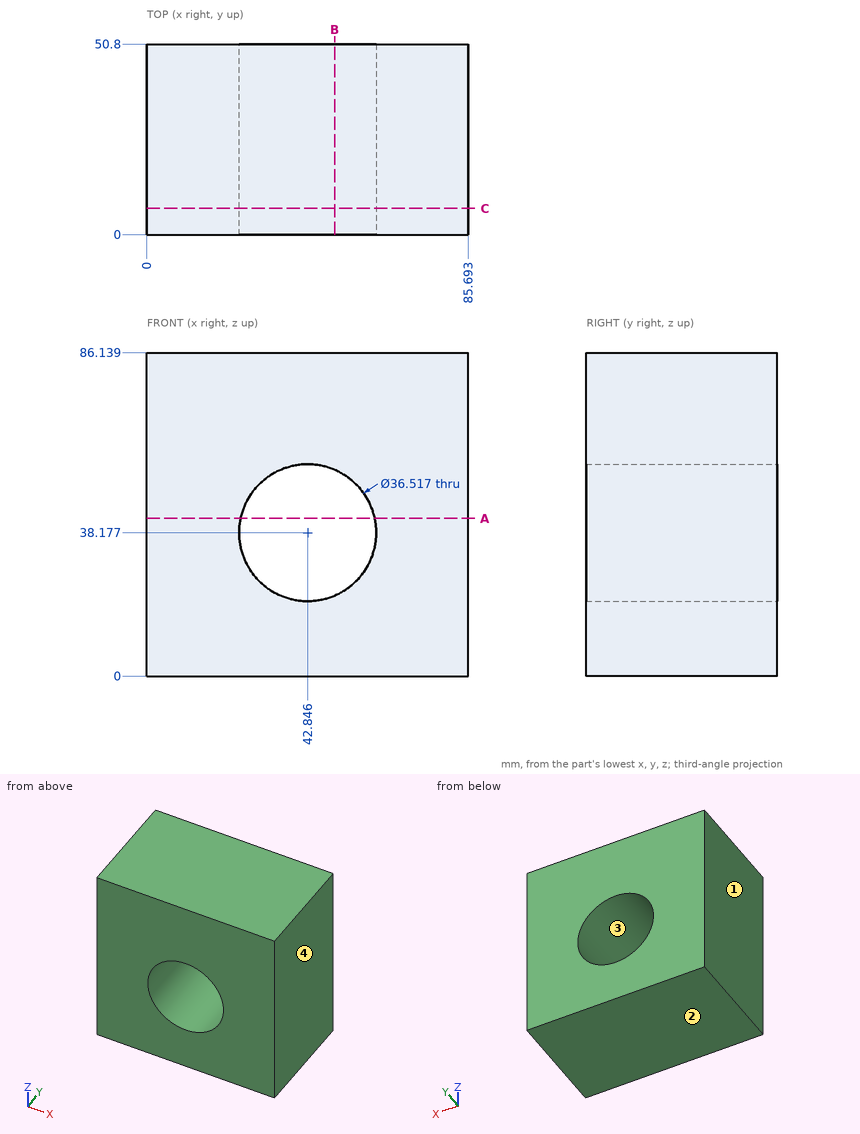
Print and shaded views of the part. All mm, measured from the part's lowest x, y and z. Coordinates: 2 decimals unless noted, no trailing zeros. Loops run counter-clockwise (first coordinate to the right, second up) from the corner with the lowest first, then second, coordinate; pieces in that order, holes last. Notation, with made-up numbers: (17, 24.25) - (21, 24.25) arc R25 cw to (21, 36.25) - close; hole circle Ø3 at (31, 1). An arc over 180 degrees is marked (long way). Use one line per item in the form item = value. Start each with the question number.
1) Two-plate mould, pull along X, no slides. Class the marked faces 1, 2, 3 and 4: +X half, -X half, draft (parallel to the pull), parting line (faces both ways), or undercut.
2) Flat gauge pin, fed straight in: pin 1 (10 mm diameter, centred on x = 37.5, z = 50.5, fed in from +Y). Where does the tip first touch, or does it go through?
3) Band-saw the part on B-B (x = 50). Give the cut face in (y, z) (1 decimal).
4) Band-saw the part on A-A (z = 42). Give the cut face in (x, y).
5) Band-saw the part on C-C (y = 7). Give the cut face in (x, z) (1 decimal), and give its area (3 significant figures).
6) Drill centre lines: L1, parallel to Z at x = 49, y = 20; L2, parallel to Z at x = 32, y = 3 (1 decimal); L3, parallel to X at y = 33, z = 29.5. Where is each one in solid material? Low to high. Write a range as from..to.
Check values:
q1.face_1 = -X half
q1.face_2 = draft
q1.face_3 = undercut
q1.face_4 = +X half
q2.pin_1 = 50.8
q3.outline = (0, 0) - (50.8, 0) - (50.8, 21.4) - (0, 21.4) - close; (0, 55) - (50.8, 55) - (50.8, 86.1) - (0, 86.1) - close
q4.outline = (0, 0) - (24.99, 0) - (24.99, 50.8) - (0, 50.8) - close; (60.7, 0) - (85.69, 0) - (85.69, 50.8) - (60.7, 50.8) - close
q5.outline = (0, 0) - (85.7, 0) - (85.7, 86.1) - (0, 86.1) - close; hole circle Ø36.5 at (42.8, 38.2)
q5.area = 6,330 mm2
q6.L1 = 0..20.99, 55.37..86.14
q6.L2 = 0..23.5, 52.9..86.1
q6.L3 = 0..26.78, 58.91..85.69
